from build123d import *

# Parameters (mm, degrees)
BOSS_EXTRUDE1_DEPTH = 10
BOSS_EXTRUDE2_DEPTH = 5
SKETCH3_R           = 10
BOSS_EXTRUDE3_DEPTH = 10


with BuildPart() as part:
    # Sketch1 → Boss-Extrude1 (new body)
    with BuildSketch(Plane.XY):
        Polygon((-45, -27.5), (-15, -27.5), (-15, -17.5), (15, -17.5), (15, -27.5), (45, -27.5), (45, -7.5), (-45, -7.5), align=None)
    extrude(amount=BOSS_EXTRUDE1_DEPTH)


with BuildPart() as body_2:
    # Sketch2 → Boss-Extrude2 (new, symmetric)
    with BuildSketch(Plane(origin=(0, 0, 0), x_dir=(0, 0, -1), z_dir=(1, 0, 0))):
        Polygon((0, -27.5), (-50, -27.5), (-50, 7.5), (-30, 7.5), (-10, -7.5), (0, -7.5), align=None)
    extrude(amount=BOSS_EXTRUDE2_DEPTH, both=True)


with BuildPart() as body_3:
    # Sketch3 → Boss-Extrude3 (new body)
    with BuildSketch(Plane.XY):
        with BuildLine():
            Line((-45, -27.5), (-15, -27.5))
            Line((-15, -27.5), (-15, -17.5))
            Line((-15, -17.5), (15, -17.5))
            Line((15, -17.5), (15, -27.5))
            Line((15, -27.5), (45, -27.5))
            Line((45, -27.5), (45, 7.5))
            Line((45, 7.5), (20, 7.5))
            ThreePointArc((20, 7.5), (0, 27.5), (-20, 7.5))
            Line((-20, 7.5), (-45, 7.5))
            Line((-45, 7.5), (-45, -27.5))
        make_face()
        with Locations((0, 7.5)):
            Circle(SKETCH3_R, mode=Mode.SUBTRACT)
    extrude(amount=-BOSS_EXTRUDE3_DEPTH)


with BuildPart() as body_3_1:
    # Body-Move/Copy1: moved
    add(body_3.part.moved(Location((0, 0, 50))))


with BuildPart() as body_2_1:
    # Body-Move/Copy2: moved
    add(body_2.part.moved(Location((40, 0, 0))))


with BuildPart() as body_4:
    # Body-Move/Copy3: copy of body 2
    add(body_2_1.part.moved(Location((-80, 0, 0))))


with BuildPart() as body_2_2:
    add(body_2_1.part)

    # Combine1: union body 3, body 4, part
    add(body_3_1.part)
    add(body_4.part)
    add(part.part)


with BuildPart() as body_2_3:
    # Body-Move/Copy5: moved
    add(body_2_2.part.moved(Location((0, 0, -25))))


solid = body_2_3.part
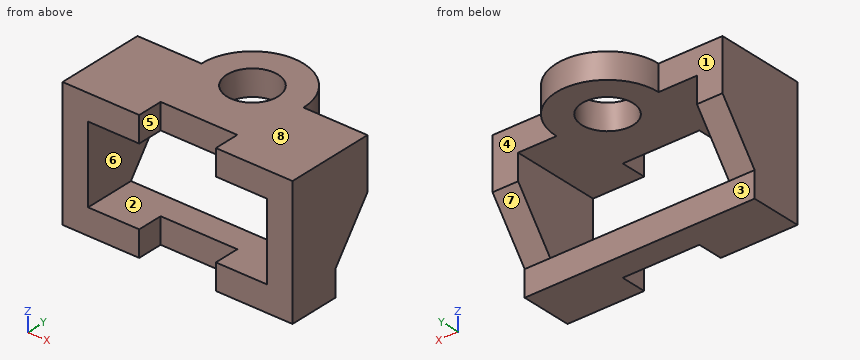
For this review, take the finished solid that the model builds, in its own axes (mm). Face numbers are marked on the shaded views. A direction names the side the tool comes from. Give positions to 0.01 mm unless a question says otherwise; leave off trailing zeros. Loops run counter-clockwise (first coordinate to the right, second up) from the corner with the lowest first, then second, coordinate; pieces in that order, holes last.
Item 1: Tool access review of the marked faces 1, 2, 3, 4 and 5: name each direction out of +Z, -Z, +X, -X, +Y, -Y from which nothing blocks a thin tool from reaching the whole face with its end or side.
Item 2: Take a section at C-C, the plane z = 14. State the section outline as (x, y) points.
Item 3: Take a section at A-A, the plane y = -11.5. State the section outline as (x, z) points, and give its area (3 significant figures).
Item 4: Take a section at D-D, the plane y = -20.5. State the section outline as (x, z) points, and give its area (3 significant figures).
Item 5: Draft analysis for pull direction Z (two halves, no side actions). For the marked faces 6, 7 and 8, state which applies: +Z half, -Z half, draft (parallel to the pull), parting line (faces both ways), or undercut.
Item 6: Insertion check: pin 1 (3 mm diameter, centred on x = 11.5, y = 9, fed in from -Z); pin 2 (6 mm diameter, centred on x = 6.5, z = 10.5, fed in from +Y); pin 3 (10 mm diameter, centred on x = -36, z = 12, fed in from +Y); pin 4 (10 mm diameter, centred on y = 17.5, z = 14, fed in from +X). Each pin has a flat end and moves straight along its axis. Give the tip position at first contact, or say it passes through.
Item 7: For line 1 along X through (y, z) = (-15, 10); line 2 along Z through (x, y) = (9, -9); line 3 along Y through (x, z) = (0, 18.5), list the stretches that pass through material, from the lowest coordinate up.
Item 8: Take a section at B-B, the plane x = 0. State the section outline as (y, z) points.
Calculated:
1. face 1: +Z, -Z, -X, +Y
1. face 2: +Y, -Y
1. face 3: -Z, +X, -X, +Y
1. face 4: +Z, -Z, +X, +Y
1. face 5: +Z, -Z, -Y
2. outline: (-45, -27.5) - (-35, -27.5) - (-35, 7.5) - (-45, 7.5) - close; (35, -27.5) - (45, -27.5) - (45, 7.5) - (35, 7.5) - close
3. outline: (-45, -25) - (45, -25) - (45, 25) - (-45, 25) - close; hole (-35, -15) - (35, -15) - (35, 15) - (-35, 15) - close
3. area: 2,400 mm2
4. outline: (-45, -25) - (-15, -25) - (-15, -15) - (-35, -15) - (-35, 15) - (-15, 15) - (-15, 25) - (-45, 25) - close; (15, -25) - (45, -25) - (45, 25) - (15, 25) - (15, 15) - (35, 15) - (35, -15) - (15, -15) - close
4. area: 1,800 mm2
5. face 6: undercut
5. face 7: -Z half
5. face 8: +Z half
6. pin 1: stops at z = 15
6. pin 2: passes through
6. pin 3: stops at y = 7.5
6. pin 4: stops at x = 19.34
7. line 1: x = -45 to -35, 35 to 45
7. line 2: z = -25 to -15, 15 to 25
7. line 3: y = -17.5 to -2.5, 17.5 to 27.5
8. outline: (-17.5, -25) - (-7.5, -25) - (-7.5, -15) - (-17.5, -15) - close; (-17.5, 15) - (-2.5, 15) - (-2.5, 25) - (-17.5, 25) - close; (17.5, 15) - (27.5, 15) - (27.5, 25) - (17.5, 25) - close
